from build123d import *

# Parameters (mm, degrees)
F0_R     = 11
F0_R_2   = 7.5
F1_DEPTH = 3
F0_R_3   = 4
F2_DEPTH = 3.75
F3_DEPTH = 6
F4_R     = 1


with BuildPart() as f1:
    # F0 (on Top) → F1 (new body)
    with BuildSketch(Plane.XY):
        Circle(F0_R)
        Circle(F0_R_2, mode=Mode.SUBTRACT)
    extrude(amount=F1_DEPTH)

    # F0 (on Top) → F2 (join)
    with BuildSketch(Plane.XY):
        Circle(F0_R_2)
        Circle(F0_R_3, mode=Mode.SUBTRACT)
    extrude(amount=F2_DEPTH)

    # F0 (on Top) → F3 (join)
    with BuildSketch(Plane.XY):
        Circle(F0_R_3)
    extrude(amount=F3_DEPTH)

    # F4
    f4_edges = [f1.edges().sort_by_distance(p)[0] for p in [
        (-11, 0, 0),
        (-11, 0, 3),
    ]]
    fillet(f4_edges, radius=F4_R)


solid = f1.part
Here's how the part is built. I have some questions about the finished solid (model axes, mm). A direction names the side the tool comes from. Round coordinates to 2 decimals unless told otherwise and drop trailing zeros. Loops run counter-clockwise (first coordinate to the right, second up) from the corner with the lowest first, then second, coordinate; pieces in that order, holes last.
1. Which directions (+Z, -Z, +X, -X, +Y, -Y) give clear straight access to the entire face, cutting with the end or side of a thin tool? Please do faces 1 (the face through (-2.38, -10.74, 1.49)), 2 (the face through (3, -3, 3.75)).
Answer list:
face 1: +Z, -Z
face 2: +Z
2. For P1, Ø1.5, axis at y = -3.5, z = 1.5, coming from the -X side; P2, Ø1.5, axis at y = 7, z = 1, coming from the -X side, each with a flat end and sliding along its axis, tell me the tip position at first contact or that it passes through.
Answer list:
P1: stops at x = -10.65
P2: stops at x = -9.05
3. If we section it at C-C on z = 1.45: Write out the boundary of the cut face in (x, y), plus the area to 3 significant figures.
Answer list:
outline: circle Ø22 at (0, 0)
area: 380 mm2
4. If I drill on line 1 along Z through (x, y) = (-5.25, 7.25); line 2 along Z through (x, y) = (-1, -4.75); line 3 along Y through (x, z) = (0.75, 3.55), over which ranges is the centre line in solid material (lowest first)?
Answer list:
line 1: z = 0 to 3
line 2: z = 0 to 3.75
line 3: y = -7.46 to 7.46
5. If we section it at A-A on x = 0: Write out the boundary of the cut face in (y, z), plus the area to 3 significant figures.
Answer list:
outline: (-11, 1) arc R1 ccw to (-10, 0) - (10, 0) arc R1 ccw to (11, 1) - (11, 2) arc R1 ccw to (10, 3) - (7.5, 3) - (7.5, 3.75) - (4, 3.75) - (4, 6) - (-4, 6) - (-4, 3.75) - (-7.5, 3.75) - (-7.5, 3) - (-10, 3) arc R1 ccw to (-11, 2) - close
area: 94.4 mm2
